Geometry check sheet. Reference: the model listing, model coordinates, mm. Round coordinates to 2 decimals unless told otherwise and drop trailing zeros. Write each loop counter-clockwise with the first axis right and the second up, starting at its lowest first coordinate (ties: lowest second). Pieces come first, ordered by that corner, then holes. Notation, with made-up numbers: M 85.5,10.25 L 104.5,10.25 A27 cw 104.5,37.25 Z; hole C 39.25,7 d10. An arc over 180 degrees is marked long. Use a Markdown table: item, result.
```python
from build123d import *

# Parameters (mm, degrees)
F1_DEPTH    = 32.766
F2_T1_DEPTH = 555.7105242514
F3_DEPTH    = 3.81
F4_T1_DEPTH = 59.0353369856


# Not quite as in the source:
# - a fillet or chamfer that OpenCascade refuses, or shapes differently, is made with other operations: its cross-section is extruded or revolved along the edge and cut away or added


with BuildPart() as f1:
    # F0 (on Front) → F1 (new body)
    with BuildSketch(Plane.XZ):
        Polygon((57.8652285039, 0), (57.8652285039, 62.5251382589), (-64.6729022264, -5.3159417585), align=None)
    extrude(amount=F1_DEPTH)

    # F2: fillet of radius 77.8169467068 on 1 edges, made by hand

    # F2_s2 → F2_t1 (cut)
    with BuildSketch(Plane.XZ.offset(-261.4722621257)):
        with BuildLine():
            ThreePointArc((57.8652285039, 0), (14.0628423673, 20.9577145427), (-33.6365297354, 11.8667997855))
            Line((-33.6365297354, 11.8667997855), (-34.3903529504, 13.228394967))
            Line((-34.3903529504, 13.228394967), (57.111405289, 63.8867334405))
            Line((57.111405289, 63.8867334405), (59.4215674381, 62.5251382589))
            ThreePointArc((59.4215674381, 62.5251382589), (59.4215674381, 31.2625691295), (58.9414404538, 1.1242591859))
            Line((58.9414404538, 1.1242591859), (57.8652285039, 0))
        make_face()
    extrude(amount=F2_T1_DEPTH, mode=Mode.SUBTRACT)

    # F3 (add): a face of the model
    f3_faces = [f1.faces().sort_by_distance(p)[0] for p in [
        (-3.4038368613, -16.383, -2.6579708792),
    ]]
    extrude(f3_faces, amount=F3_DEPTH)

    # F4: chamfer of 5.08 on 1 edges, made by hand

    # F4_s2 → F4_t1 (cut)
    with BuildSketch(Plane.XZ.offset(-13.1346684928)):
        Polygon((-60.2285595639, -2.8554096417), (-64.4527290592, -10.3911682338), (-64.6729022264, -5.3159417585), align=None)
    extrude(amount=F4_T1_DEPTH, mode=Mode.SUBTRACT)


solid = f1.part
```
Item 1: Cross-section at B-B, the plane z = 14.5. Record the cut outline in (x, y), and give its area (3 significant figures).
Outcome:
| item | result |
|---|---|
| outline | M -28.43,-32.77 L 36.54,-32.77 L 36.54,0 L -28.43,0 Z |
| area | 2,130 mm2 |
Item 2: Cross-section at C-C, the plane x = -53. Record the cut outline in (y, z), and give its area (3 significant figures).
Outcome:
| item | result |
|---|---|
| outline | M -32.77,-8.62 L 0,-8.62 L 0,1.15 L -32.77,1.15 Z |
| area | 320 mm2 |
Item 3: Material ranges on line 1 along X through (y, z) = (-5.5, 9.5); line 2 along X through (y, z) = (-9, 2) (3 decimals); line 3 along Z through (x, y) = (-9.5, -24), recorded low to high. Write a range as from..to.
Outcome:
| item | result |
|---|---|
| line 1 | x = -37.91..45.74 |
| line 2 | x = -51.458..55.695 |
| line 3 | z = -6.74..20.41 |
Item 4: Go/stop test with flat-tipped pins: pin 1 (6 mm diameter, centred on y = -27, z = 3.5, fed in from +X); pin 2 (1.5 mm diameter, centred on x = -21.5, y = -24, fed in from -Z). Record where each tip stops, or that it passes through.
Outcome:
| item | result |
|---|---|
| pin 1 | stops at x = 57.34 |
| pin 2 | stops at z = -7.29 |
Item 5: Cross-section at A-A, the plane y = -23. Record the cut outline in (x, z), and give its area (3 significant figures).
Outcome:
| item | result |
|---|---|
| outline | M -63.72,-9.09 L 58.03,-3.81 L 57.87,0 A77.82 ccw -33.64,11.87 L -60.23,-2.86 Z |
| area | 2,380 mm2 |
